Drawing for the job (mm, zero at the part's lowest x, y, z). Round coordinates to 2 decimals unless told otherwise and drop trailing zeros. Order: outer loops, then holes, each group sorted by start corner. A loop starts at its lowest first (then second) coordinate and runs counter-clockwise, first axis right, second up. Notation, with made-up numbers: (-11, 38.25) - (-1, 38.25) arc R18 ccw to (-1, 48.25) - close; hole circle Ø6 at (40.5, 9.5). An arc over 180 degrees is marked (long way). Answer as a JSON object with one key per item and string values.
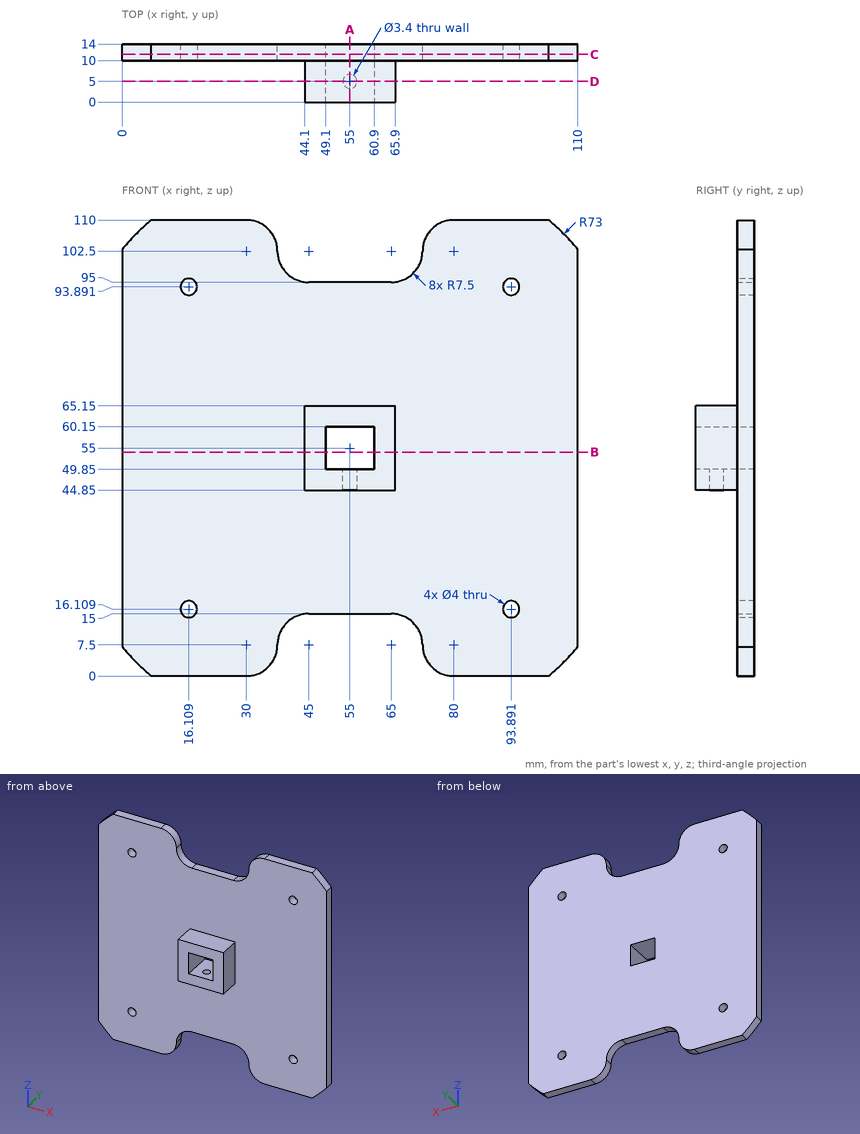
Item 1: Cut at A-A (x = 55). Write the cut outline in (y, z), plus the area to 3 significant figures.
Taken from the geometry:
{"outline": "(0, 44.85) - (3.3, 44.85) - (3.3, 49.85) - (0, 49.85) - close; (0, 60.15) - (14, 60.15) - (14, 95) - (10, 95) - (10, 65.15) - (0, 65.15) - close; (6.7, 44.85) - (10, 44.85) - (10, 15) - (14, 15) - (14, 49.85) - (6.7, 49.85) - close", "area": "362 mm2"}
Item 2: Probe L1, parallel to Z at x = 60, y = 0.5; L2, parallel to X at y = 1, z = 60; L3, parallel to Z at x = 15, y = 10.75 (1 decimal). List the from-to ranges inside material, lowest first. Write a range as from..to.
Taken from the geometry:
{"L1": "44.85..49.85, 60.15..65.15", "L2": "44.1..49.1, 60.9..65.9", "L3": "0..14.4, 17.8..92.2, 95.6..110"}
Item 3: Cut at B-B (z = 54). Write the cut outline in (x, y).
Taken from the geometry:
{"outline": "(0, 10) - (44.1, 10) - (44.1, 0) - (49.1, 0) - (49.1, 14) - (0, 14) - close; (60.9, 0) - (65.9, 0) - (65.9, 10) - (110, 10) - (110, 14) - (60.9, 14) - close"}
Item 4: Cut at D-D (y = 5). Write the cut outline in (x, z).
Taken from the geometry:
{"outline": "(44.1, 44.85) - (53.3, 44.85) - (53.3, 49.85) - (49.1, 49.85) - (49.1, 60.15) - (60.9, 60.15) - (60.9, 49.85) - (56.7, 49.85) - (56.7, 44.85) - (65.9, 44.85) - (65.9, 65.15) - (44.1, 65.15) - close"}
Item 5: Cut at C-C (y = 11.5). Write the cut outline in (x, z).
Taken from the geometry:
{"outline": "(0, 7) arc R73 ccw to (7, 0) - (30, 0) arc R7.5 ccw to (37.5, 7.5) arc R7.5 cw to (45, 15) - (65, 15) arc R7.5 cw to (72.5, 7.5) arc R7.5 ccw to (80, 0) - (103, 0) arc R73 ccw to (110, 7) - (110, 103) arc R73 ccw to (103, 110) - (80, 110) arc R7.5 ccw to (72.5, 102.5) arc R7.5 cw to (65, 95) - (45, 95) arc R7.5 cw to (37.5, 102.5) arc R7.5 ccw to (30, 110) - (7, 110) arc R73 ccw to (0, 103) - close; hole circle Ø4 at (16.11, 16.11); hole circle Ø4 at (16.11, 93.89); hole (49.1, 49.85) - (60.9, 49.85) - (60.9, 60.15) - (49.1, 60.15) - close; hole circle Ø4 at (93.89, 16.11); hole circle Ø4 at (93.89, 93.89)"}
Item 6: Drop flat-ended pins along their axis: P1, Ø3, axis at x = 59.5, y = 12, coming from the +Z side; P2, Ø5, axis at x = 93.89, z = 93.89, coming from the +Y side; P3, Ø4.5, axis at x = 55, y = 5, coming from the -Z side; P4, Ø10, axis at x = 73.5, z = 86.5, coming from the -Y side. Give the stop position or say it passes through.
Taken from the geometry:
{"P1": "z = 95", "P2": "y = 14", "P3": "z = 44.85", "P4": "y = 10"}
